from build123d import *

# Parameters (mm, degrees)
SKETCH2_R             = 0.940847183
BOSS_EXTRUDE1_DEPTH   = 2
SKETCH2_R_2           = 1.25
BOSS_EXTRUDE1_2_DEPTH = 2
BOSS_EXTRUDE3_DEPTH   = 3
SKETCH2_7_R           = 1.25
SKETCH2_7_R_2         = 0.940847183
BOSS_EXTRUDE4_DEPTH   = 8.5
SKETCH3_R             = 1.6
BOSS_EXTRUDE5_DEPTH   = 1.5
FILLET3_R             = 1
FILLET4_R             = 1
FILLET5_R             = 1
SKETCH4_W             = 22.082114238
SKETCH4_H             = 4.26025432
CUT_EXTRUDE1_DEPTH    = 10
FILLET6_R             = 1
FILLET7_R             = 1


with BuildPart() as part:
    # Sketch2 → Boss-Extrude1 (new body)
    with BuildSketch(Plane.XY.offset(5)):
        with Locations((45.192420188, 1.674673151)):
            Circle(SKETCH2_R)
    extrude(amount=BOSS_EXTRUDE1_DEPTH)


with BuildPart() as body_2:
    # Sketch2 → Boss-Extrude1 2 (new body)
    with BuildSketch(Plane.XY.offset(5)):
        with BuildLine():
            Line((41.133082748, 37.634349985), (34.706148145, 42.236237142))
            ThreePointArc((34.706148145, 42.236237142), (31.067550303, 43.449692764), (27.378275076, 42.400351494))
            Line((27.378275076, 42.400351494), (20.830773346, 38.142250332))
            ThreePointArc((20.830773346, 38.142250332), (19.658086914, 37.165968028), (18.745312064, 35.94319958))
            Line((18.745312064, 35.94319958), (7.704226172, 16.81947026))
            ThreePointArc((7.704226172, 16.81947026), (7.101694806, 15.417636125), (6.842562909, 13.91396274))
            Line((6.842562909, 13.91396274), (6.421786289, 5.985399395))
            ThreePointArc((6.421786289, 5.985399395), (7.283504465, 2.390948015), (9.965555118, -0.152522691))
            Line((9.965555118, -0.152522691), (17.042257133, -3.752468769))
            ThreePointArc((17.042257133, -3.752468769), (18.474071457, -4.279870659), (19.989385244, -4.458949249))
            Line((19.989385244, -4.458949249), (42.071499482, -4.458949249))
            ThreePointArc((42.071499482, -4.458949249), (43.586809148, -4.279873865), (45.018620578, -3.752477043))
            Line((45.018620578, -3.752477043), (52.023196139, -0.18925451))
            ThreePointArc((52.023196139, -0.18925451), (54.750476182, 2.433850072), (55.55467988, 6.131415554))
            Line((55.55467988, 6.131415554), (54.945383885, 13.619853326))
            ThreePointArc((54.945383885, 13.619853326), (54.671858346, 15.028435929), (54.095948871, 16.342684554))
            Line((54.095948871, 16.342684554), (42.978078812, 35.599415021))
            ThreePointArc((42.978078812, 35.599415021), (42.164300135, 36.715454096), (41.133082748, 37.634349985))
        make_face()
        with Locations((45.192420188, 1.674673151)):
            Circle(SKETCH2_R_2, mode=Mode.SUBTRACT)
        Polygon((21.92114362, 34.943199877), (39.968717021, 34.943199877), (40.676589536, 3.339551379), (15.692425848, 3.937560139), (15.692425848, 20.422570873), (19.971987097, 20.422570873), (19.971987097, 30.940834749), (21.92114362, 30.940834749), align=None, mode=Mode.SUBTRACT)
    extrude(amount=BOSS_EXTRUDE1_2_DEPTH)

    # Sketch2<4> → Boss-Extrude3 (add)
    with BuildSketch(Plane.XY.offset(5)):
        with BuildLine():
            Line((41.133082748, 37.634349985), (34.706148145, 42.236237142))
            ThreePointArc((34.706148145, 42.236237142), (31.067550303, 43.449692764), (27.378275076, 42.400351494))
            Line((27.378275076, 42.400351494), (20.830773346, 38.142250332))
            ThreePointArc((20.830773346, 38.142250332), (19.658086914, 37.165968028), (18.745312064, 35.94319958))
            Line((18.745312064, 35.94319958), (7.704226172, 16.81947026))
            ThreePointArc((7.704226172, 16.81947026), (7.101694806, 15.417636125), (6.842562909, 13.91396274))
            Line((6.842562909, 13.91396274), (6.421786289, 5.985399395))
            ThreePointArc((6.421786289, 5.985399395), (7.283504465, 2.390948015), (9.965555118, -0.152522691))
            Line((9.965555118, -0.152522691), (17.042257133, -3.752468769))
            ThreePointArc((17.042257133, -3.752468769), (18.474071457, -4.279870659), (19.989385244, -4.458949249))
            Line((19.989385244, -4.458949249), (42.071499482, -4.458949249))
            ThreePointArc((42.071499482, -4.458949249), (43.586809148, -4.279873865), (45.018620578, -3.752477043))
            Line((45.018620578, -3.752477043), (52.023196139, -0.18925451))
            ThreePointArc((52.023196139, -0.18925451), (54.750476182, 2.433850072), (55.55467988, 6.131415554))
            Line((55.55467988, 6.131415554), (54.945383885, 13.619853326))
            ThreePointArc((54.945383885, 13.619853326), (54.671858346, 15.028435929), (54.095948871, 16.342684554))
            Line((54.095948871, 16.342684554), (42.978078812, 35.599415021))
            ThreePointArc((42.978078812, 35.599415021), (42.164300135, 36.715454096), (41.133082748, 37.634349985))
        make_face()
        with BuildLine():
            Line((42.071514619, -2.458949249), (19.989371788, -2.458949249))
            ThreePointArc((19.989371788, -2.458949249), (18.940310927, -2.334974581), (17.949056442, -1.969854112))
            Line((17.949056442, -1.969854112), (10.872362442, 1.630087888))
            ThreePointArc((10.872362442, 1.630087888), (9.015554367, 3.390949582), (8.41897619, 5.8794159))
            Line((8.41897619, 5.8794159), (8.839752837, 13.807979751))
            ThreePointArc((8.839752837, 13.807979751), (9.019149806, 14.848983048), (9.436284279, 15.819482904))
            Line((9.436284279, 15.819482904), (20.477363044, 34.943199877))
            ThreePointArc((20.477363044, 34.943199877), (21.109284015, 35.789731503), (21.92114362, 36.465618987))
            Line((21.92114362, 36.465618987), (28.468652286, 40.72372466))
            ThreePointArc((28.468652286, 40.72372466), (31.022767484, 41.450194202), (33.54179906, 40.610109469))
            Line((33.54179906, 40.610109469), (39.968717021, 36.008234228))
            ThreePointArc((39.968717021, 36.008234228), (40.682635911, 35.37207361), (41.24601974, 34.599429336))
            Line((41.24601974, 34.599429336), (52.363900573, 15.342680208))
            ThreePointArc((52.363900573, 15.342680208), (52.762607381, 14.432817969), (52.951972413, 13.457647575))
            Line((52.951972413, 13.457647575), (53.561268099, 5.969213602))
            ThreePointArc((53.561268099, 5.969213602), (53.004512325, 3.409355177), (51.116390771, 1.593357064))
            Line((51.116390771, 1.593357064), (44.111826917, -1.969859513))
            ThreePointArc((44.111826917, -1.969859513), (43.120573578, -2.334976851), (42.071514619, -2.458949249))
        make_face(mode=Mode.SUBTRACT)
    extrude(amount=BOSS_EXTRUDE3_DEPTH)

    # Sketch2<7> → Boss-Extrude4 (add)
    with BuildSketch(Plane.XY.offset(5)):
        with Locations((45.192420188, 1.674673151)):
            Circle(SKETCH2_7_R)
        with Locations((45.192420188, 1.674673151)):
            Circle(SKETCH2_7_R_2, mode=Mode.SUBTRACT)
        with Locations((17.192425388, 1.674673151)):
            Circle(SKETCH2_7_R)
        with Locations((17.192425388, 1.674673151)):
            Circle(SKETCH2_7_R_2, mode=Mode.SUBTRACT)
    extrude(amount=BOSS_EXTRUDE4_DEPTH)

    # Sketch3 → Boss-Extrude5 (add)
    with BuildSketch(Plane(origin=(0, 0, 5), x_dir=(-1, 0, 0), z_dir=(0, 0, -1))):
        with BuildLine():
            Line((-57.465912559, 7.334344298), (-61.7249195, 7.560353667))
            ThreePointArc((-61.7249195, 7.560353667), (-64.727209986, 10.899141147), (-61.388422506, 13.901431633))
            Line((-61.388422506, 13.901431633), (-56.679353565, 13.651539178))
            ThreePointArc((-56.679353565, 13.651539178), (-55.433923512, 14.005056034), (-54.665941639, 15.047300739))
            Line((-54.665941639, 15.047300739), (-55.572883446, 5.399998251))
            ThreePointArc((-55.572883446, 5.399998251), (-56.142498996, 6.736019854), (-57.465912559, 7.334344298))
        make_face()
        with Locations((-61.556671003, 10.73089265)):
            Circle(SKETCH3_R, mode=Mode.SUBTRACT)
        with BuildLine():
            Line((-17.846979662, 44.100626478), (-20.486080778, 40.282409595))
            ThreePointArc((-20.486080778, 40.282409595), (-20.824333172, 38.888857435), (-20.142867401, 37.627109954))
            Line((-20.142867401, 37.627109954), (-28.341017566, 42.916928771))
            ThreePointArc((-28.341017566, 42.916928771), (-26.996383012, 42.829749498), (-25.901618076, 43.615327019))
            Line((-25.901618076, 43.615327019), (-23.070638788, 47.711150724))
            ThreePointArc((-23.070638788, 47.711150724), (-18.653547102, 48.517718164), (-17.846979662, 44.100626478))
        make_face()
        with Locations((-20.458809225, 45.905888601)):
            Circle(SKETCH3_R, mode=Mode.SUBTRACT)
        with BuildLine():
            Line((-13.224518296, -8.670350201), (-15.108259251, -4.967291533))
            ThreePointArc((-15.108259251, -4.967291533), (-16.179685102, -4.004819306), (-17.619913769, -4.011713354))
            Line((-17.619913769, -4.011713354), (-8.938003872, 0.497808514))
            ThreePointArc((-8.938003872, 0.497808514), (-9.666330862, -0.646021526), (-9.497643296, -1.991514696))
            Line((-9.497643296, -1.991514696), (-7.564735193, -5.791226163))
            ThreePointArc((-7.564735193, -5.791226163), (-8.955064726, -10.060679733), (-13.224518296, -8.670350201))
        make_face()
        with Locations((-10.394626745, -7.230788182)):
            Circle(SKETCH3_R, mode=Mode.SUBTRACT)
    extrude(amount=-BOSS_EXTRUDE5_DEPTH)

    # Fillet3
    fillet3_edges = [body_2.edges().sort_by_distance(p)[0] for p in [
        (15.942425388, 1.674673151, 7),
        (43.942420188, 1.674673151, 7),
    ]]
    fillet(fillet3_edges, radius=FILLET3_R)

    # Fillet4
    fillet4_edges = [body_2.edges().sort_by_distance(p)[0] for p in [
        (19.971987097, 20.422570873, 6),
        (15.692425848, 20.422570873, 6),
        (15.692425848, 3.937560139, 6),
        (40.676589536, 3.339551379, 6),
        (39.968717021, 34.943199877, 6),
        (21.92114362, 34.943199877, 6),
        (21.92114362, 30.940834749, 6),
    ]]
    fillet(fillet4_edges, radius=FILLET4_R)

    # Fillet5
    fillet5_edges = [body_2.edges().sort_by_distance(p)[0] for p in [
        (19.971987097, 30.940834749, 6),
    ]]
    fillet(fillet5_edges, radius=FILLET5_R)

    # Sketch4 → Cut-Extrude1 (cut)
    with BuildSketch(Plane.XZ.offset(4.458949249)):
        with Locations((31.030442363, 5.86987284)):
            Rectangle(SKETCH4_W, SKETCH4_H)
    extrude(amount=-CUT_EXTRUDE1_DEPTH, mode=Mode.SUBTRACT)

    # Fillet6
    fillet6_edges = [body_2.edges().sort_by_distance(p)[0] for p in [
        (19.989385244, 3.834710214, 6),
        (40.627279379, 5.541050751, 6),
    ]]
    fillet(fillet6_edges, radius=FILLET6_R)

    # Fillet7
    fillet7_edges = [body_2.edges().sort_by_distance(p)[0] for p in [
        (42.071499482, 5.541050751, 6),
    ]]
    fillet(fillet7_edges, radius=FILLET7_R)


with BuildPart() as part_1:
    add(part.part)

    # Combine1: union body 2
    add(body_2.part)


solid = part_1.part
Design review of the part built by this model. Coordinates are the model's own, in mm. A direction names the side the tool comes from. Round coordinates to 2 decimals unless told otherwise and drop trailing zeros. Write each loop counter-clockwise with the first axis right and the second up, starting at its lowest first coordinate (ties: lowest second). Pieces come first, ordered by that corner, then holes. Notation, with made-up numbers: (71.25, 52) - (117.25, 52) arc R24 ccw to (117.25, 64) - close; hole circle Ø9 at (53.25, 44.25). An arc over 180 degrees is marked (long way). Use a Markdown table: item, result. Add a question column.
1. Wall thickness on probe 1 along X at (y, z) = (1.5, 9); probe 2 along Z at (x, y) = (50.5, 15); probe 3 along Z at (x, y) = (24, 39): over which ranges is each line inside the solid? List them lowest first.
2. Mouldability with a two-part tool opening along Y and no side actions: class faces 5 (the face through (41, 16, 7)), 6 (the face through (9.034, 3.36, 7.493)), 7 (the face through (18.453, -4.275, 6.479)), 8 (the face through (37.965, 39.903, 6.479)) as +Y half, -Y half, draft (parallel to the pull), parting line (faces both ways), or undercut.
3. Clearance check with flat-ended pins moving along their axes: pin 1 (2 mm diameter, centred on x = 17.5, z = 6.5, fed in from -Y); pin 2 (1 mm diameter, centred on x = 48, y = 5.5, fed in from +Z); pin 3 (3 mm diameter, centred on x = 51.5, z = 8, fed in from -Y). State where each tip first meets the part, or that it passes through.
4. We need section A-A (y = 18.5). State the section outline as (x, z) points, then the cut area to 3 significant figures.
5. We need section B-B (z = 9.25). State the section outline as (x, y) points, then the cut area to 3 significant figures.
6. For faces 1 (the face through (55.254, 9.823, 7.24)), 2 (the face through (40.674, 35.382, 7.493)), 3 (the face through (18, 20.423, 6)), 4 (the face through (22, 43, 6.5)), list the 3-axis set-ups (+Z, -Z, +X, -X, +Y, -Y) from which the entire face can be reached by the end or side of a thin tool; tool diameter is ignored.
Output:
| question | item | result |
|---|---|---|
| 1 | probe 1 | x = 15.95 to 16.27, 18.12 to 18.43, 43.95 to 44.27, 46.12 to 46.43 |
| 1 | probe 2 | z = 5 to 7 |
| 1 | probe 3 | z = 5 to 8 |
| 2 | face 5 | undercut |
| 2 | face 6 | undercut |
| 2 | face 7 | -Y half |
| 2 | face 8 | +Y half |
| 3 | pin 1 | stops at y = -4.29 |
| 3 | pin 2 | stops at z = 7 |
| 3 | pin 3 | stops at y = -1.22 |
| 4 | outline | (8.67, 5) - (15.69, 5) - (15.69, 7) - (10.98, 7) - (10.98, 8) - (8.67, 8) - close; (40.34, 5) - (52.85, 5) - (52.85, 8) - (50.54, 8) - (50.54, 7) - (40.34, 7) - close |
| 4 | area | 43.7 mm2 |
| 5 | outline | circle Ø2.5 at (17.19, 1.67); circle Ø2.5 at (45.19, 1.67); hole circle Ø1.88 at (17.19, 1.67); hole circle Ø1.88 at (45.19, 1.67) |
| 5 | area | 4.26 mm2 |
| 6 | face 1 | +Z, +X, +Y |
| 6 | face 2 | +Z, -Y |
| 6 | face 3 | +Z, -Z |
| 6 | face 4 | +Z, -X, +Y |
